Here's how the part is built. I have some questions about the finished solid (model axes, mm). Face numbers are marked on the shaded views. A direction names the side the tool comes from. Give positions to 0.01 mm unless a question says otherwise; leave off trailing zeros. Loops run counter-clockwise (first coordinate to the right, second up) from the corner with the lowest first, then second, coordinate; pieces in that order, holes last. Notation, with made-up numbers: M -2.75,-35.75 L 35.25,-35.75 A16 cw 35.25,-6.75 Z; hole C -19,52.5 d10. An arc over 180 degrees is marked long. Answer as CSV lines item,"result". Start each with the question number.
Item 1: For the marked faces 1 and 2, which set-ups out of +Z, -Z, +X, -X, +Y, -Y let a thin tool reach every point of the face, with its end or its side?
Item 2: If I drill on line 1 along X through (y, z) = (32, 15.5); line 2 along Y through (x, z) = (20, 17.75); line 3 along X through (y, z) = (-12, 10), over which ranges is the centre line in solid material (lowest first)? Write a range as from..to.
Item 3: Will these pins go through, and if not, where does the flat tip stop? P1, Ø1.3, axis at y = 1.51, z = 11.6, coming from the +X side; P2, Ø2, axis at y = 25, z = 9.5, coming from the +X side; P3, Ø0.9, axis at y = -13.5, z = 20.5, coming from the +X side; P4, Ø3, axis at x = 19.89, z = 11.6, coming from the +Y side.
Item 4: I want a section at B-B on y = 15. List the corners of the cut face in (x, z) for me, plus the area to 3 significant figures.
Item 5: I want a section at A-A on z = 11.6. Give the number of separate pieces and of enclosed holes in the cut face, plus the area to 3 significant figures.
Item 6: I want a section at D-D on x = -3.5. List the corners of the cut face in (y, z) for me.
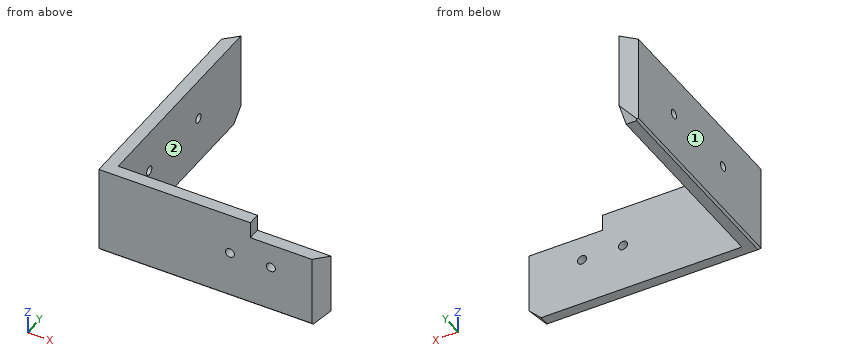
from build123d import *

# Parameters (mm, degrees)
F1_DEPTH  = 21.6
F2_W      = 52
F2_H      = 52
F3_DEPTH  = 22
F4_SIZE   = 2.99999
F5_SIZE   = 0.5
F6_R      = 1.1
F7_DEPTH  = 3
F8_R      = 1.1
F9_DEPTH  = 3
F10_W     = 18
F10_H     = 4
F11_DEPTH = 3


# Not quite as in the source:
# - a fillet or chamfer is up to 0.001 mm smaller than in the source, because OpenCascade refuses the exact size


with BuildPart() as f1:
    # F0 (on Top) → F1 (new body)
    with BuildSketch(Plane.XY):
        Polygon((-12.1071431786, 40.3610856729), (-12.1071431786, -14.6389143271), (42.8928568214, -14.6389143271), (42.8928568214, 7.8610856729), (10.3928568214, 40.3610856729), align=None)
    extrude(amount=F1_DEPTH)

    # F2 (on face) → F3 (cut)
    with BuildSketch(Plane.XY.offset(21.6)):
        with Locations((16.8928568214, 14.3610856729)):
            Rectangle(F2_W, F2_H)
    extrude(amount=-F3_DEPTH, mode=Mode.SUBTRACT)

    # F4 (size 3 in the source; OpenCascade refuses exactly that, so slightly less here)
    f4_edges = [f1.edges().sort_by_distance(p)[0] for p in [
        (42.892857, -13.138914, 0),
        (-10.607143, 40.361086, 0),
        (-12.107143, 40.361086, 10.8),
        (42.892857, -14.638914, 10.8),
    ]]
    chamfer(f4_edges, length=F4_SIZE)

    # F5
    f5_edges = [f1.edges().sort_by_distance(p)[0] for p in [
        (13.892862, -14.638914, 0),
        (-12.107143, 11.361091, 0),
    ]]
    chamfer(f5_edges, length=F5_SIZE)

    # F6 (on face) → F7 (cut)
    with BuildSketch(Plane.XZ.offset(14.6389143271)):
        with Locations((29.8928568214, 11.6)):
            Circle(F6_R)
        with Locations((19.8928568214, 11.6)):
            Circle(F6_R)
    extrude(amount=-F7_DEPTH, mode=Mode.SUBTRACT)

    # F8 (on face) → F9 (cut)
    with BuildSketch(Plane(origin=(-12.1071431786, 0, 0), x_dir=(0, -1, 0), z_dir=(-1, 0, 0))):
        with Locations((-22.3610856729, 11.6)):
            Circle(F8_R)
        with Locations((-1.5111208195, 11.6)):
            Circle(F8_R)
    extrude(amount=-F9_DEPTH, mode=Mode.SUBTRACT)

    # F10 (on face) → F11 (cut)
    with BuildSketch(Plane(origin=(0, -11.6389143271, 0), x_dir=(-1, 0, 0), z_dir=(0, 1, 0))):
        with Locations((-33.8928568214, 19.6)):
            Rectangle(F10_W, F10_H)
    extrude(amount=-F11_DEPTH, mode=Mode.SUBTRACT)


solid = f1.part
Result:
1,face 1,"+Z, -Z, -X, +Y, -Y"
1,face 2,"+Z, -Z, +X, +Y"
2,line 1,"-12.11..-9.11"
2,line 2,"-14.64..-11.64"
2,line 3,"-12.11..42.53"
3,P1,"through"
3,P2,"x = -9.11"
3,P3,"x = 24.89"
3,P4,"y = -11.64"
4,outline,"M -12.11,0.5 L -11.61,0 L -9.11,0 L -9.11,21.6 L -12.11,21.6 Z"
4,area,"64.7 mm^2"
5,separate pieces,"5"
5,enclosed holes,"0"
5,area,"286 mm^2"
6,outline,"M -14.64,0.5 L -14.14,0 L -11.64,0 L -11.64,21.6 L -14.64,21.6 Z"
